For this review, take the finished solid that the model builds, in its own axes (mm). Round coordinates to 2 decimals unless told otherwise and drop trailing zeros. Write each loop counter-clockwise with the first axis right and the second up, starting at its lowest first coordinate (ties: lowest second). Pieces come first, ordered by that corner, then holes. Notation, with made-up numbers: (28, -4.75) - (36, -4.75) arc R6 ccw to (36, 6.25) - close; hole circle Ø3 at (-37, 32). An arc over 180 degrees is marked (long way). One line per item, written item: value. Start each with the question number.
Q1. For probe 1 along Y at (x, z) = (0, -4); probe 2 along Y at (x, z) = (3, -5); probe 3 along X at (y, z) = (-10, -3.75), list the stretches that pass through material, from the lowest coordinate up.
Q2. Clearance check with a flat-ended pin moving along its axis: pin 1 Ø3 at (x, y) = (26.94, -9.06) entering from -Z. State where the tip first meets the part, or that it passes through.
Q3. Add section B-B on x = 26.94. Write out the cut boundary in (y, z), and give its area (3 significant figures).
Q4. Add section D-D on z = -4. Give the number of separate pieces and of enclosed holes in the cut face, and give its area (3 significant figures).
Q5. Add section A-A on y = 26.5. Write out the cut boundary in (x, z), and give its area (3 significant figures).
Q6. Add section C-C on y = 85. Write out the cut boundary in (x, z) (3 decimals).
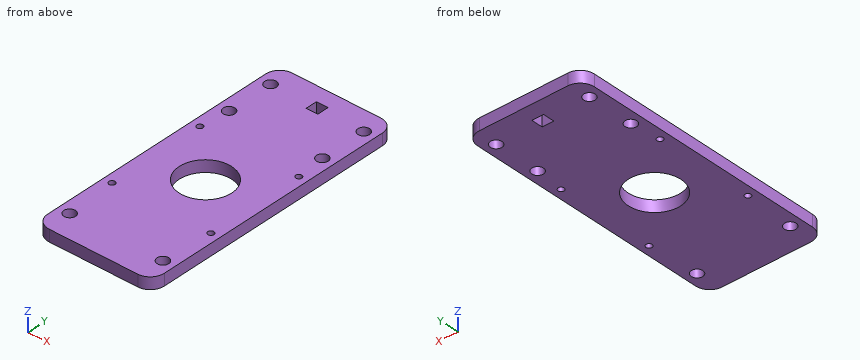
```python
from build123d import *

# Parameters (mm, degrees)
BOSS_EXTRUDE1_DEPTH = 6.35
SKETCH2_R           = 1.35
SKETCH2_R_2         = 1.385
CUT_EXTRUDE1_DEPTH  = 38.116505762
SKETCH3_W           = 63.5
SKETCH3_H           = 88.9
SKETCH3_W_2         = 38.321076004
SKETCH3_H_2         = 47.237540142
BOSS_EXTRUDE2_DEPTH = 6.35
SKETCH5_W           = 27.94
SKETCH5_H           = 55.88
CUT_EXTRUDE3_DEPTH  = 61.153053743
SKETCH6_R           = 3.175
CUT_EXTRUDE4_DEPTH  = 61.153053743
SKETCH7_W           = 41.724968974
SKETCH7_H           = 57.858351452
BOSS_EXTRUDE3_DEPTH = 6.35
SKETCH8_R           = 14.2875
CUT_EXTRUDE5_DEPTH  = 6.35
SKETCH10_W          = 63.5
SKETCH10_H          = 60
SKETCH10_R          = 3.175
SKETCH10_W_2        = 6.33
SKETCH10_H_2        = 6.33
BOSS_EXTRUDE4_DEPTH = 6.35
FILLET1_R           = 7.62
SKETCH11_R          = 1.65
CUT_EXTRUDE6_DEPTH  = 104.404858197


with BuildPart() as part:
    # Sketch1 → Boss-Extrude1 (new body)
    with BuildSketch(Plane.XY):
        with BuildLine():
            Line((-19.69889026, 23.2987845), (-14.850045261, 29.75147823))
            ThreePointArc((-14.850045261, 29.75147823), (-14.144755454, 30.339267512), (-13.251155001, 30.55))
            Line((-13.251155001, 30.55), (13.251155001, 30.55))
            ThreePointArc((13.251155001, 30.55), (14.144755454, 30.339267512), (14.850045261, 29.75147823))
            Line((14.850045261, 29.75147823), (19.69889026, 23.2987845))
            ThreePointArc((19.69889026, 23.2987845), (19.997074131, 22.730638521), (20.1, 22.09730627))
            Line((20.1, 22.09730627), (20.1, -22.09730627))
            ThreePointArc((20.1, -22.09730627), (19.997074131, -22.730638521), (19.69889026, -23.2987845))
            Line((19.69889026, -23.2987845), (14.850045261, -29.75147823))
            ThreePointArc((14.850045261, -29.75147823), (14.144755454, -30.339267512), (13.251155001, -30.55))
            Line((13.251155001, -30.55), (-13.251155001, -30.55))
            ThreePointArc((-13.251155001, -30.55), (-14.144755454, -30.339267512), (-14.850045261, -29.75147823))
            Line((-14.850045261, -29.75147823), (-19.69889026, -23.2987845))
            ThreePointArc((-19.69889026, -23.2987845), (-19.997074131, -22.730638521), (-20.1, -22.09730627))
            Line((-20.1, -22.09730627), (-20.1, 22.09730627))
            ThreePointArc((-20.1, 22.09730627), (-19.997074131, 22.730638521), (-19.69889026, 23.2987845))
        make_face()
    extrude(amount=-BOSS_EXTRUDE1_DEPTH)

    # Sketch2 → Cut-Extrude1 (cut, through all)
    with BuildSketch(Plane(origin=(0, 0, -6.35), x_dir=(-1, 0, 0), z_dir=(0, 0, -1))):
        with Locations((17.3, 21.9487845)):
            Circle(SKETCH2_R)
        with Locations((17.3, -0.0512155)):
            Circle(SKETCH2_R)
        with Locations((17.3, -22.0512155)):
            Circle(SKETCH2_R)
        with Locations((11, -27.75)):
            Circle(SKETCH2_R_2)
        with Locations(Location((-11, -27.75, 0), (0, 0, 180))):
            Circle(SKETCH2_R_2)
        with Locations(Location((-17.3, -22.0512155, 0), (0, 0, 180))):
            Circle(SKETCH2_R)
        with Locations(Location((-17.3, -0.0512155, 0), (0, 0, 180))):
            Circle(SKETCH2_R)
        with Locations(Location((-17.3, 21.9487845, 0), (0, 0, 180))):
            Circle(SKETCH2_R)
    extrude(amount=-CUT_EXTRUDE1_DEPTH, mode=Mode.SUBTRACT)

    # Sketch3 → Boss-Extrude2 (add)
    with BuildSketch(Plane(origin=(0, 0, -6.35), x_dir=(-1, 0, 0), z_dir=(0, 0, -1))):
        with Locations((0, -6.2452155)):
            Rectangle(SKETCH3_W, SKETCH3_H)
        Rectangle(SKETCH3_W_2, SKETCH3_H_2, mode=Mode.SUBTRACT)
    extrude(amount=-BOSS_EXTRUDE2_DEPTH)

    # Sketch5 → Cut-Extrude3 (cut, through all)
    with BuildSketch(Plane.XY):
        with Locations((0, 3.0087845)):
            Rectangle(SKETCH5_W, SKETCH5_H)
    extrude(amount=-CUT_EXTRUDE3_DEPTH, mode=Mode.SUBTRACT)

    # Sketch6 → Cut-Extrude4 (cut, through all)
    with BuildSketch(Plane(origin=(0, 0, -6.35), x_dir=(-1, 0, 0), z_dir=(0, 0, -1))):
        with Locations((-25.4, -36.7252155)):
            Circle(SKETCH6_R)
        with Locations((25.4, -36.7252155)):
            Circle(SKETCH6_R)
    extrude(amount=-CUT_EXTRUDE4_DEPTH, mode=Mode.SUBTRACT)

    # Sketch7 → Boss-Extrude3 (add)
    with BuildSketch(Plane(origin=(0, 0, -6.35), x_dir=(-1, 0, 0), z_dir=(0, 0, -1))):
        with Locations((0, 3.16744248)):
            Rectangle(SKETCH7_W, SKETCH7_H)
    extrude(amount=-BOSS_EXTRUDE3_DEPTH)

    # Sketch8 → Cut-Extrude5 (cut)
    with BuildSketch(Plane(origin=(0, 0, -6.35), x_dir=(-1, 0, 0), z_dir=(0, 0, -1))):
        with Locations((0, 17.8847845)):
            Circle(SKETCH8_R)
    extrude(amount=-CUT_EXTRUDE5_DEPTH, mode=Mode.SUBTRACT)

    # Sketch10 → Boss-Extrude4 (add)
    with BuildSketch(Plane(origin=(0, 0, -6.35), x_dir=(-1, 0, 0), z_dir=(0, 0, -1))):
        with Locations((0, 68.2047845)):
            Rectangle(SKETCH10_W, SKETCH10_H)
        with Locations((-25.4, 86.3797845)):
            Circle(SKETCH10_R, mode=Mode.SUBTRACT)
        with Locations((-25.4, 60.9797845)):
            Circle(SKETCH10_R, mode=Mode.SUBTRACT)
        with Locations(Location((25.4, 60.9797845, 0), (0, 0, 180))):
            Circle(SKETCH10_R, mode=Mode.SUBTRACT)
        with Locations(Location((25.4, 86.3797845, 0), (0, 0, 180))):
            Circle(SKETCH10_R, mode=Mode.SUBTRACT)
        with Locations((0, 86.3797845)):
            Rectangle(SKETCH10_W_2, SKETCH10_H_2, mode=Mode.SUBTRACT)
    extrude(amount=-BOSS_EXTRUDE4_DEPTH)

    # Fillet1
    fillet1_edges = [part.edges().sort_by_distance(p)[0] for p in [
        (31.75, 98.2047845, -3.175),
        (-31.75, 98.2047845, -3.175),
        (-31.75, -50.6952155, -3.175),
        (31.75, -50.6952155, -3.175),
    ]]
    fillet(fillet1_edges, radius=FILLET1_R)

    # Sketch11 → Cut-Extrude6 (cut, through all)
    with BuildSketch(Plane.XY):
        with Locations((-26.94, 44.8247845)):
            Circle(SKETCH11_R)
        with Locations((26.94, 44.8247845)):
            Circle(SKETCH11_R)
        with Locations((-26.94, -9.055983818)):
            Circle(SKETCH11_R)
        with Locations((26.94, -9.055983818)):
            Circle(SKETCH11_R)
    extrude(amount=-CUT_EXTRUDE6_DEPTH, mode=Mode.SUBTRACT)


solid = part.part
```
Result set:
1. probe 1: y = -50.7 to 3.6, 32.17 to 83.21, 89.54 to 98.2
1. probe 2: y = -50.7 to 3.92, 31.85 to 83.21, 89.54 to 98.2
1. probe 3: x = -31.75 to -28.29, -25.59 to 25.59, 28.29 to 31.75
2. pin 1: passes through
3. outline: (-50.16, -6.35) - (-39.5, -6.35) - (-39.5, 0) - (-50.16, 0) - close; (-33.95, -6.35) - (-10.71, -6.35) - (-10.71, 0) - (-33.95, 0) - close; (-7.41, -6.35) - (43.17, -6.35) - (43.17, 0) - (-7.41, 0) - close; (46.47, -6.35) - (58.2, -6.35) - (58.2, 0) - (46.47, 0) - close; (63.76, -6.35) - (83.6, -6.35) - (83.6, 0) - (63.76, 0) - close; (89.16, -6.35) - (97.67, -6.35) - (97.67, 0) - (89.16, 0) - close
3. area: 791 mm^2
4. separate pieces: 1
4. enclosed holes: 12
4. area: 8,500 mm^2
5. outline: (-31.75, -6.35) - (-11.4, -6.35) - (-11.4, 0) - (-31.75, 0) - close; (11.4, -6.35) - (31.75, -6.35) - (31.75, 0) - (11.4, 0) - close
5. area: 258 mm^2
6. outline: (-31.75, -6.35) - (-28.26, -6.35) - (-28.26, 0) - (-31.75, 0) - close; (-22.54, -6.35) - (-3.165, -6.35) - (-3.165, 0) - (-22.54, 0) - close; (3.165, -6.35) - (22.54, -6.35) - (22.54, 0) - (3.165, 0) - close; (28.26, -6.35) - (31.75, -6.35) - (31.75, 0) - (28.26, 0) - close
